Geometry check sheet. Reference: the model listing, model coordinates, mm. Give positions to 0.01 mm unless a question says otherwise; leave off trailing zeros. Order: outer loops, then holes, each group sorted by start corner. A loop starts at its lowest first (then second) coordinate and runs counter-clockwise, first axis right, second up. Notation, with made-up numbers: M 89,-5 L 117,-5 A23 cw 117,11 Z; hole C 52.5,-6 d4. An arc over 180 degrees is marked long. Answer as CSV lines item,"result". Start each with the question number.
Q1. Section check D-D, the plane x = -44.45. Record the boundary of the cut face in (y, z) (1 decimal), then the cut area to 3 significant figures.
Q2. Section check C-C, the plane x = -171.45. Record the boundary of the cut face in (y, z) (1 decimal), then the cut area to 3 significant figures.
Q3. Section check B-B, the plane y = 82.55. Record the boundary of the cut face in (x, z) (1 decimal), then the cut area to 3 significant figures.
Q4. Thickness scan on line 1 (X direction, y = 82.5, z = 2.25); line 2 (X direction, y = 10.5, z = 1); line 3 (X direction, y = 82, z = 1.5). Record the ranges inside material, lowest first.
Q5. Section check A-A, the plane y = 20.32. Record the boundary of the cut face in (x, z) (1 decimal), then the cut area to 3 significant figures.
Q6. Go/stop test with flat-tipped pins: pin 1 (1 mm diameter, centred on x = -120, z = 0.5, fed in from -Y); pin 2 (1 mm diameter, centred on y = -2, z = 1, fed in from +X). Record where each tip stops, or that it passes through.
```python
from build123d import *

# Parameters (mm, degrees)
BOSS_EXTRUDE1_DEPTH = 3.175
SKETCH2_R           = 1.5875
CUT_EXTRUDE1_DEPTH  = 3.175
BOSS_EXTRUDE2_DEPTH = 3.175
CUT_EXTRUDE2_DEPTH  = 3.175
SKETCH5_W           = 1.5875
SKETCH5_H           = 12.7
CUT_EXTRUDE3_DEPTH  = 10.16
LPATTERN1_COUNT     = 2
LPATTERN1_PITCH     = 25.4
SKETCH8_W           = 38.1
SKETCH8_H           = 46.355
CUT_EXTRUDE6_DEPTH  = 12.7
SKETCH10_R          = 1.5875
CUT_EXTRUDE7_DEPTH  = 7.62
CUT_EXTRUDE8_DEPTH  = 12.7
FILLET1_R           = 25.4
SKETCH13_W          = 25.4
SKETCH13_H          = 177.8
BOSS_EXTRUDE3_DEPTH = 3.175
LPATTERN2_COUNT     = 2
LPATTERN2_PITCH     = 76.2
SKETCH14_W          = 19.05
SKETCH14_H          = 6.35
BOSS_EXTRUDE4_DEPTH = 3.175
FILLET2_R           = 1.905
CUT_EXTRUDE9_DEPTH  = 392.916423648
SKETCH16_R          = 3.2385
CUT_EXTRUDE10_DEPTH = 205.735785414
SKETCH17_R          = 1.75
CUT_EXTRUDE11_DEPTH = 205.735785414
SKETCH18_W          = 33.274
SKETCH18_H          = 6.35
CUT_EXTRUDE12_DEPTH = 205.735785414


with BuildPart() as part:
    # Sketch1 → Boss-Extrude1 (new body)
    with BuildSketch(Plane.XY):
        Polygon((0, 0), (-177.8, 0), (-177.8, 349.25), (-25.4, 349.25), align=None)
    extrude(amount=BOSS_EXTRUDE1_DEPTH)

    # Sketch2 → Cut-Extrude1 (cut)
    with BuildSketch(Plane.XY.offset(3.175)):
        with Locations((-127, 133.35)):
            Circle(SKETCH2_R)
        with Locations((-127, 306.07)):
            Circle(SKETCH2_R)
    extrude(amount=-CUT_EXTRUDE1_DEPTH, mode=Mode.SUBTRACT)

    # Sketch3 → Boss-Extrude2 (add)
    with BuildSketch(Plane.XY.offset(3.175)):
        Polygon((-63.5, 88.9), (63.5, 111.29352655), (63.5, 187.49352655), (-63.5, 187.49352655), align=None)
    extrude(amount=-BOSS_EXTRUDE2_DEPTH)

    # Sketch4 → Cut-Extrude2 (cut)
    with BuildSketch(Plane.XY.offset(3.175)):
        Polygon((-44.45, 110.49), (-31.942941537, 112.695331856), (-32.494274501, 115.822096472), (-45.001332964, 113.616764616), align=None)
        Polygon((-6.92882461, 117.105995569), (5.578233853, 119.311327425), (5.026900889, 122.438092041), (-7.480157574, 120.232760185), align=None)
    cut_extrude2 = extrude(amount=-CUT_EXTRUDE2_DEPTH, mode=Mode.SUBTRACT)

    # Sketch5 → Cut-Extrude3 (cut)
    with BuildSketch(Plane.XY.offset(3.175)):
        with Locations((-126.20625, 209.55)):
            Rectangle(SKETCH5_W, SKETCH5_H)
        with Locations((-127.79375, 209.55)):
            Rectangle(SKETCH5_W, SKETCH5_H)
    cut_extrude3 = extrude(amount=-CUT_EXTRUDE3_DEPTH, mode=Mode.SUBTRACT)

    # LPattern1: Cut-Extrude3 ×2
    with Locations(*[(0, i * LPATTERN1_PITCH, 0) for i in range(1, LPATTERN1_COUNT)]):
        add(cut_extrude3, mode=Mode.SUBTRACT)

    # Sketch8 → Cut-Extrude6 (cut)
    with BuildSketch(Plane.XY.offset(3.175)):
        with Locations((-19.05, 23.1775)):
            Rectangle(SKETCH8_W, SKETCH8_H)
    extrude(amount=-CUT_EXTRUDE6_DEPTH, mode=Mode.SUBTRACT)

    # Sketch10 → Cut-Extrude7 (cut)
    with BuildSketch(Plane(origin=(0, 0, 0), x_dir=(-1, 0, 0), z_dir=(0, 0, -1))):
        with Locations((171.45, 20.32)):
            Circle(SKETCH10_R)
        with Locations((44.45, 20.32)):
            Circle(SKETCH10_R)
    extrude(amount=-CUT_EXTRUDE7_DEPTH, mode=Mode.SUBTRACT)

    # Sketch11 → Cut-Extrude8 (cut)
    with BuildSketch(Plane(origin=(0, 0, 0), x_dir=(-1, 0, 0), z_dir=(0, 0, -1))):
        with BuildLine():
            Line((62.738, 18.199261314), (62.738, 5.499261314))
            ThreePointArc((62.738, 5.499261314), (65.913, 6.35), (69.088, 5.499261314))
            Line((69.088, 5.499261314), (69.088, 18.199261314))
            Line((69.088, 18.199261314), (62.738, 18.199261314))
        make_face()
        with BuildLine():
            Line((69.088, 5.499261314), (62.738, 5.499261314))
            ThreePointArc((62.738, 5.499261314), (60.413738686, 3.175), (59.563, 0))
            Line((59.563, 0), (72.263, 0))
            ThreePointArc((72.263, 0), (71.412261314, 3.175), (69.088, 5.499261314))
        make_face()
        with BuildLine():
            ThreePointArc((153.543, 5.499261314), (151.218738686, 3.175), (150.368, 0))
            Line((150.368, 0), (163.068, 0))
            ThreePointArc((163.068, 0), (162.217261314, 3.175), (159.893, 5.499261314))
            Line((159.893, 5.499261314), (153.543, 5.499261314))
        make_face()
        with BuildLine():
            Line((153.543, 18.199261314), (153.543, 5.499261314))
            ThreePointArc((153.543, 5.499261314), (156.718, 6.35), (159.893, 5.499261314))
            Line((159.893, 5.499261314), (159.893, 18.199261314))
            Line((159.893, 18.199261314), (153.543, 18.199261314))
        make_face()
        with BuildLine():
            ThreePointArc((159.893, 5.499261314), (156.718, 6.35), (153.543, 5.499261314))
            Line((153.543, 5.499261314), (159.893, 5.499261314))
        make_face()
    extrude(amount=-CUT_EXTRUDE8_DEPTH, mode=Mode.SUBTRACT)


with BuildPart() as cut_extrude8_kept_piece:
    # of the separate pieces the step leaves, the one the design keeps (cut_extrude8_pieces_kept)
    add(part.part.solids().sort_by_distance((-38.1, 0, 0))[0])

    # Fillet1
    fillet1_edges = [cut_extrude8_kept_piece.edges().sort_by_distance(p)[0] for p in [
        (-38.1, 46.355, 1.5875),
    ]]
    fillet(fillet1_edges, radius=FILLET1_R)

    # Sketch13 → Boss-Extrude3 (add)
    with BuildSketch(Plane(origin=(0, 0, 0), x_dir=(-1, 0, 0), z_dir=(0, 0, -1))):
        with Locations((12.7, 260.35)):
            Rectangle(SKETCH13_W, SKETCH13_H)
    extrude(amount=-BOSS_EXTRUDE3_DEPTH)

    # LPattern2: Cut-Extrude2 ×2
    with Locations(*[Vector(0.9848077530122078, 0.17364817766693205, 0) * (i * LPATTERN2_PITCH) for i in range(1, LPATTERN2_COUNT)]):
        add(cut_extrude2, mode=Mode.SUBTRACT)

    # Sketch14 → Boss-Extrude4 (add)
    with BuildSketch(Plane(origin=(0, 0, 0), x_dir=(-1, 0, 0), z_dir=(0, 0, -1))):
        with Locations((85.725, -3.175)):
            Rectangle(SKETCH14_W, SKETCH14_H)
        with Locations((136.525, -3.175)):
            Rectangle(SKETCH14_W, SKETCH14_H)
    extrude(amount=-BOSS_EXTRUDE4_DEPTH)

    # Fillet2
    fillet2_edges = [cut_extrude8_kept_piece.edges().sort_by_distance(p)[0] for p in [
        (-153.543, 5.499261314, 1.5875),
        (-153.543, 18.199261314, 1.5875),
        (-159.893, 18.199261314, 1.5875),
        (-159.893, 5.499261314, 1.5875),
        (-62.738, 5.499261314, 1.5875),
        (-62.738, 18.199261314, 1.5875),
        (-69.088, 18.199261314, 1.5875),
        (-69.088, 5.499261314, 1.5875),
    ]]
    fillet(fillet2_edges, radius=FILLET2_R)

    # Sketch15 → Cut-Extrude9 (cut, through all)
    with BuildSketch(Plane(origin=(0, 0, 0), x_dir=(-1, 0, 0), z_dir=(0, 0, -1))):
        Polygon((38.1, 20.955), (38.1, 38.915512242), (59.646092876, 38.915512242), (59.646092876, 87.95072106), (59.646092876, 101.458470342), (177.8, 101.458470342), (320.979610432, 349.25), (0, 416.848504921), (-115.466676424, 312.716348385), (-102.18599125, 94.704595701), align=None)
    extrude(amount=-CUT_EXTRUDE9_DEPTH, mode=Mode.SUBTRACT)

    # Sketch16 → Cut-Extrude10 (cut, through all)
    with BuildSketch(Plane.XY.offset(3.175)):
        with Locations((-131.064, 82.55)):
            Circle(SKETCH16_R)
    extrude(amount=-CUT_EXTRUDE10_DEPTH, mode=Mode.SUBTRACT)

    # Sketch17 → Cut-Extrude11 (cut, through all)
    with BuildSketch(Plane.XY.offset(3.175)):
        with Locations((-122.682, 82.55)):
            Circle(SKETCH17_R)
        with Locations(Location((-139.446, 82.55, 0), (0, 0, 180))):
            Circle(SKETCH17_R)
    extrude(amount=-CUT_EXTRUDE11_DEPTH, mode=Mode.SUBTRACT)

    # Sketch18 → Cut-Extrude12 (cut, through all)
    with BuildSketch(Plane(origin=(0, 0, 0), x_dir=(-1, 0, 0), z_dir=(0, 0, -1))):
        with Locations((111.125, -3.175)):
            Rectangle(SKETCH18_W, SKETCH18_H)
    extrude(amount=-CUT_EXTRUDE12_DEPTH, mode=Mode.SUBTRACT)


solid = cut_extrude8_kept_piece.part
```
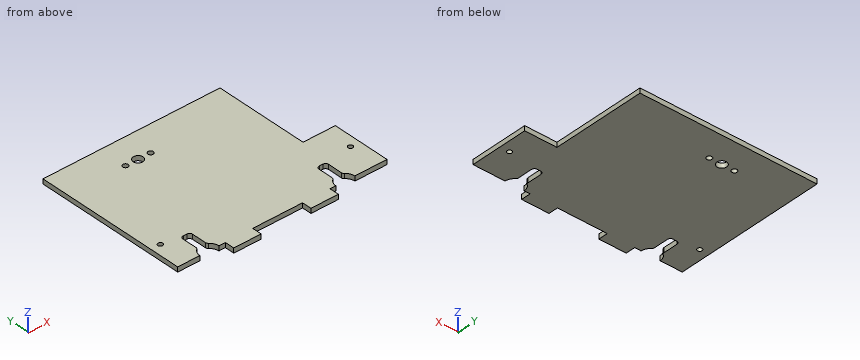
Answer block:
1,outline,"M 0,0 L 18.7,0 L 18.7,3.2 L 0,3.2 Z; M 21.9,0 L 38.9,0 L 38.9,3.2 L 21.9,3.2 Z"
1,area,"113 mm2"
2,outline,"M 0,0 L 18.7,0 L 18.7,3.2 L 0,3.2 Z; M 21.9,0 L 101.5,0 L 101.5,3.2 L 21.9,3.2 Z"
2,area,"312 mm2"
3,outline,"M -177.8,0 L -141.2,0 L -141.2,3.2 L -177.8,3.2 Z; M -137.7,0 L -134.3,0 L -134.3,3.2 L -137.7,3.2 Z; M -127.8,0 L -124.4,0 L -124.4,3.2 L -127.8,3.2 Z; M -120.9,0 L -59.6,0 L -59.6,3.2 L -120.9,3.2 Z"
3,area,"332 mm2"
4,line 1,"x = -177.8 to -141.2, -137.7 to -134.3, -127.83 to -124.43, -120.93 to -59.65"
4,line 2,"x = -177.8 to -159.89, -153.54 to -69.09, -62.74 to -38.1"
4,line 3,"x = -177.8 to -141.11, -137.78 to -134.26, -127.87 to -124.34, -121.02 to -59.65"
5,outline,"M -177.8,0 L -173,0 L -173,3.2 L -177.8,3.2 Z; M -169.9,0 L -46,0 L -46,3.2 L -169.9,3.2 Z; M -42.9,0 L -38.1,0 L -38.1,3.2 L -42.9,3.2 Z"
5,area,"423 mm2"
6,pin 1,"stops at y = 0"
6,pin 2,"stops at x = -76.2"
